```python
from build123d import *

# Parameters (mm, degrees)
SKETCH1_R           = 12
BOSS_EXTRUDE1_DEPTH = 90
SKETCH3_OUTSIDE_W   = 45.238
SKETCH3_OUTSIDE_H   = 45.238
SKETCH3_OUTSIDE_R   = 9.525
CUT_EXTRUDE1_DEPTH  = 40
SKETCH4_OUTSIDE_W   = 45.238
SKETCH4_OUTSIDE_H   = 45.238
SKETCH4_OUTSIDE_R   = 9.525
CUT_EXTRUDE2_DEPTH  = 40
SKETCH6_R           = 7.15
CUT_EXTRUDE3_DEPTH  = 91
CHAMFER1_SIZE       = 1.2
CUT_EXTRUDE4_DEPTH  = 91


with BuildPart() as part:
    # Sketch1 → Boss-Extrude1 (new body)
    with BuildSketch(Plane.XY):
        Circle(SKETCH1_R)
    extrude(amount=BOSS_EXTRUDE1_DEPTH)

    # Sketch3 outside → Cut-Extrude1 (cut)
    with BuildSketch(Plane.XY.offset(90)):
        Rectangle(SKETCH3_OUTSIDE_W, SKETCH3_OUTSIDE_H)
        Circle(SKETCH3_OUTSIDE_R, mode=Mode.SUBTRACT)
    extrude(amount=-CUT_EXTRUDE1_DEPTH, mode=Mode.SUBTRACT)

    # Sketch4 outside → Cut-Extrude2 (cut)
    with BuildSketch(Plane(origin=(0, 0, 0), x_dir=(-1, 0, 0), z_dir=(0, 0, -1))):
        Rectangle(SKETCH4_OUTSIDE_W, SKETCH4_OUTSIDE_H)
        Circle(SKETCH4_OUTSIDE_R, mode=Mode.SUBTRACT)
    extrude(amount=-CUT_EXTRUDE2_DEPTH, mode=Mode.SUBTRACT)

    # Sketch6 → Cut-Extrude3 (cut, through all)
    with BuildSketch(Plane.XY.offset(90)):
        Circle(SKETCH6_R)
    extrude(amount=-CUT_EXTRUDE3_DEPTH, mode=Mode.SUBTRACT)

    # Chamfer1
    chamfer1_edges = [part.edges().sort_by_distance(p)[0] for p in [
        (-7.15, 0, 90),
    ]]
    chamfer(chamfer1_edges, length=CHAMFER1_SIZE)

    # Sketch7 → Cut-Extrude4 (cut, through all)
    with BuildSketch(Plane(origin=(0, 0, 0), x_dir=(-1, 0, 0), z_dir=(0, 0, -1))):
        Polygon((0, 11.15), (-4.435932822, 11.15), (-4.435932822, 13.87296042), (4.435932822, 13.87296042), (4.435932822, 11.15), align=None)
    extrude(amount=-CUT_EXTRUDE4_DEPTH, mode=Mode.SUBTRACT)

    # Sketch10 → Revolve1 (revolve)
    with BuildSketch(Plane(origin=(0, 0, 0), x_dir=(1, 0, 0), z_dir=(0, 1, 0))):
        with BuildLine():
            Line((9.525, 0), (14.629409523, 1.367722409))
            ThreePointArc((14.629409523, 1.367722409), (14.89667667, 1.546304608), (15, 1.850685323))
            Line((15, 1.850685323), (15, 5))
            Line((15, 5), (9, 5))
            Line((9, 5), (9, 2.5))
            Line((9, 2.5), (7.15, 2.5))
            Line((7.15, 2.5), (7.15, 0))
            Line((7.15, 0), (9.525, 0))
        make_face()
    revolve(axis=Axis((0, 0, 1.6), (0, 0, -1)))


solid = part.part
```
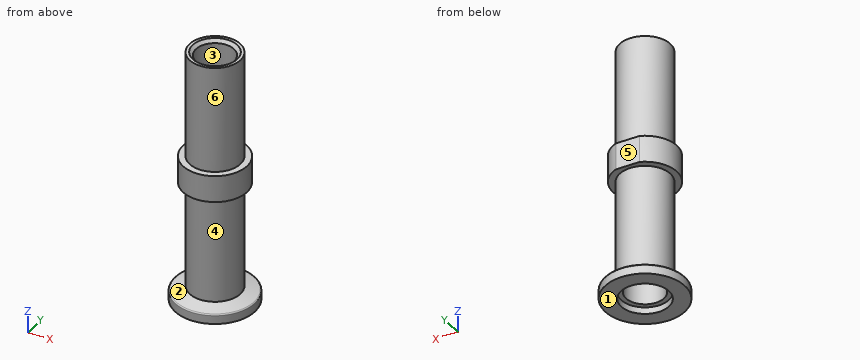
Could you check a few things on this model? Use its own coordinates, in mm. Face numbers are marked on the shaded views. A direction names the side the tool comes from. Give positions to 0.01 mm unless a question says otherwise; leave off trailing zeros. Loops run counter-clockwise (first coordinate to the right, second up) from the corner with the lowest first, then second, coordinate; pieces in that order, holes last. Notation, with made-up numbers: (5.5, -10) - (14.5, -10) arc R34 cw to (14.5, 22) - close; hole circle Ø3 at (31, -38.5). An arc over 180 degrees is marked (long way). Answer in a Markdown table with one row per item. Add a question column.
Q1. If we section it at D-D (z = 41.5): List the corners of the cut face in (x, y) for me.
Q2. If we section it at B-B (y = 0): List the corners of the cut face in (x, z) for me (3 decimals), plus the area to 3 significant figures.
Q3. If we section it at A-A (x = 0): List the corners of the cut face in (y, z) for me (3 decimals), plus the area to 3 significant figures.
Q4. For pin 1 (8 mm diameter, centred on x = -2.5, z = 10, fed in from -Y) (3 decimals); pin 2 (16.5 mm diameter, centred on x = 0, y = 0, fed in from +Z); pin 3 (12 mm diameter, centred on y = 5.5, z = 7.5, fed in from +X) (3 decimals), each with a flat end and sliding along its axis, tell me the tip position at first contact or that it passes through.
Q5. Which directions (+Z, -Z, +X, -X, +Y, -Y) give clear straight access to the entire face, cutting with the end or side of a thin tool? Please do the marked faces 4, 5 and 6.
Q6. Please list where these lines run through material, in increasing order: L1, parallel to Y at x = 0, z = -3.7; L2, parallel to Y at x = 0, z = 42. Write a range as from..to.
Q7. If we section it at C-C (z = 66): List the corners of the cut face in (x, y) for me (3 decimals).
Q8. We'd pull the mould along X, two halves only. Please class the marked faces 1, 2 and 3: +X half, -X half, draft (parallel to the pull), parting line (faces both ways), or undercut.
The answers:
| question | item | result |
|---|---|---|
| 1 | outline | (-4.44, 11.15) arc R12 ccw (long way) to (4.44, 11.15) - close; hole circle Ø14.3 at (0, 0) |
| 2 | outline | (-15, -5) - (-9, -5) - (-9, -2.5) - (-7.15, -2.5) - (-7.15, 88.8) - (-8.35, 90) - (-9.525, 90) - (-9.525, 50) - (-12, 50) - (-12, 40) - (-9.525, 40) - (-9.525, 0) - (-14.629, -1.368) arc R0.5 ccw to (-15, -1.851) - close; (7.15, -2.5) - (9, -2.5) - (9, -5) - (15, -5) - (15, -1.851) arc R0.5 ccw to (14.629, -1.368) - (9.525, 0) - (9.525, 40) - (12, 40) - (12, 50) - (9.525, 50) - (9.525, 90) - (8.35, 90) - (7.15, 88.8) - close |
| 2 | area | 537 mm^2 |
| 3 | outline | (-15, -5) - (-9, -5) - (-9, -2.5) - (-7.15, -2.5) - (-7.15, 88.8) - (-8.35, 90) - (-9.525, 90) - (-9.525, 50) - (-12, 50) - (-12, 40) - (-9.525, 40) - (-9.525, 0) - (-14.629, -1.368) arc R0.5 ccw to (-15, -1.851) - close; (7.15, -2.5) - (9, -2.5) - (9, -5) - (15, -5) - (15, -1.851) arc R0.5 ccw to (14.629, -1.368) - (9.525, 0) - (9.525, 40) - (11.15, 40) - (11.15, 50) - (9.525, 50) - (9.525, 90) - (8.35, 90) - (7.15, 88.8) - close |
| 3 | area | 528 mm^2 |
| 4 | pin 1 | stops at y = -9.525 |
| 4 | pin 2 | stops at z = 89.9 |
| 4 | pin 3 | stops at x = 9.525 |
| 5 | face 4 | none |
| 5 | face 5 | +Z, +X, -X, +Y |
| 5 | face 6 | +Z |
| 6 | L1 | y = -15..-9, 9..15 |
| 6 | L2 | y = -12..-7.15, 7.15..11.15 |
| 7 | outline | circle Ø19.05 at (0, 0); hole circle Ø14.3 at (0, 0) |
| 8 | face 1 | draft |
| 8 | face 2 | parting line |
| 8 | face 3 | undercut |
